Check sheet for the modelled part. Datum: model origin and axes. Units: mm. A direction names the side the tool comes from. Round coordinates to 2 decimals unless told otherwise and drop trailing zeros. Loops run counter-clockwise (first coordinate to the right, second up) from the corner with the lowest first, then second, coordinate; pieces in that order, holes last. Notation, with made-up numbers: (22.25, -22.5) - (59.25, -22.5) arc R24 cw to (59.25, 5.5) - close; hole circle Ø11 at (-17, 44). An arc over 180 degrees is marked (long way). Put each result on its own line as item: value. Start each with the question number.
Item 1: Gauge pin test, flat ends, axial feed: pin 1 Ø0.8 at (x, z) = (4, 97.5) entering from +Y; pin 2 Ø0.8 at (x, z) = (-3.5, 152.5) entering from -Y; pin 3 Ø1.5 at (x, y) = (-7.5, -1.5) entering from +Z (1 decimal); pin 4 Ø1.6 at (x, z) = (0.5, 215.5) entering from -Y. Record the tip position at first contact, or that the pin passes through.
Item 2: Section check C-C, the plane z = 235. Give the number of separate pieces and of enclosed holes in the cut face, and give its area (3 significant figures).
Item 3: Material ranges on line 1 along X through (y, z) = (7, 236); line 2 along Y through (x, z) = (-8.25, 139), recorded low to high.
Item 4: Section check A-A, the plane x = 0. Record the cut outline in (y, z), and give its area (3 significant figures).
Item 5: Tool access check on faces 1 (the flat face through (3.5, 0, 143)), 2 (the flat face through (0, -3.5, 143)), 3 (the flat face through (0, -3, 0)). Record the directions out of +Z, -Z, +X, -X, +Y, -Y that give a thin tool (end or side, any length) a straight path to the whole face; none if there is none.
Item 6: Draft check along X on faces 4 (the flat face through (-3.5, 0, 143)), 5 (the flat face through (0, -3, 290)), 6 (the cylindrical face through (-0.54, 2.44, 142.97)), 7 (the flat face through (0, 3.5, 143)). Enter one of: pulls with the +X half, pulls with the -X half, needs draft (parallel to the pull), parting line crosses it, or undercut.
Autodesk Inventor part; units mm, degrees
ref_plane "Начальная плоскость" through (0, 0, 0) normal (0, 0, 1) x (1, 0, 0)
ref_plane "Конечная плоскость" through (0, 0, 290) normal (0, 0, 1) x (1, 0, 0)
ref_plane "YZ Plane" through (0, 0, 0) normal (1, 0, 0) x (0, 1, 0)
ref_plane "Начальная плоскость" through (0, 0, 0) normal (0, 0, 1) x (1, 0, 0)
ref_plane "Конечная плоскость" through (0, 0, 290) normal (0, 0, 1) x (1, 0, 0)
sketch "Эскиз" plane through (0, 0, 0) normal (0, 0, 1) x (1, 0, 0)
  line L0 (-14.4349, 0) -> (14.4349, 0)
  line L1 (0, -14) -> (0, 14)
  line L2 (0, 0) -> (7.5, 7.5) construction
  circle A0 centre (7.5, 7.5) radius 1.65 construction
  line L3 (5.85, 9.15) -> (9.15, 9.15)
  line L4 (9.15, 9.15) -> (9.15, 5.85)
  line L5 (9.15, 5.85) -> (5.85, 5.85)
  line L6 (5.85, 5.85) -> (5.85, 9.15)
  line L7 (3.235, 8.1636) -> (4.72, 9.9636)
  line L8 (4.7971, 10) -> (8.5, 10)
  line L9 (3.3121, 8) -> (4.95, 8)
  line L10 (4.95, 8) -> (4.95, 5.7985)
  line L11 (4.95, 5.7985) -> (2.6515, 3.5)
  line L12 (0, 3.5) -> (2.6515, 3.5)
  circle A1 centre (0, 0) radius 2.5
  line L13 (8.1636, 3.235) -> (9.9636, 4.72)
  line L14 (10, 4.7971) -> (10, 8.5)
  line L15 (8, 3.3121) -> (8, 4.95)
  line L16 (8, 4.95) -> (5.7985, 4.95)
  line L17 (5.7985, 4.95) -> (3.5, 2.6515)
  line L18 (3.5, 0) -> (3.5, 2.6515)
  arc A2 (10, 8.5) -> (8.5, 10) centre (8.5, 8.5) ccw
  line L19 (0, 0) -> (-7.5, 7.5) construction
  circle A3 centre (-7.5, 7.5) radius 1.65 construction
  line L20 (-5.85, 9.15) -> (-9.15, 9.15)
  line L21 (-9.15, 9.15) -> (-9.15, 5.85)
  line L22 (-9.15, 5.85) -> (-5.85, 5.85)
  line L23 (-5.85, 5.85) -> (-5.85, 9.15)
  line L24 (-3.235, 8.1636) -> (-4.72, 9.9636)
  line L25 (-4.7971, 10) -> (-8.5, 10)
  line L26 (-3.3121, 8) -> (-4.95, 8)
  line L27 (-4.95, 8) -> (-4.95, 5.7985)
  line L28 (-4.95, 5.7985) -> (-2.6515, 3.5)
  line L29 (0, 3.5) -> (-2.6515, 3.5)
  line L30 (-3.5, 0) -> (-3.5, 2.6515)
  line L31 (-5.7985, 4.95) -> (-3.5, 2.6515)
  line L32 (-8, 4.95) -> (-5.7985, 4.95)
  line L33 (-8, 3.3121) -> (-8, 4.95)
  line L34 (-8.1636, 3.235) -> (-9.9636, 4.72)
  line L35 (-10, 4.7971) -> (-10, 8.5)
  arc A4 (-8.5, 10) -> (-10, 8.5) centre (-8.5, 8.5) ccw
  line L36 (0, 14) -> (0, -14)
  line L37 (0, 0) -> (7.5, -7.5) construction
  circle A5 centre (7.5, -7.5) radius 1.65 construction
  line L38 (5.85, -9.15) -> (9.15, -9.15)
  line L39 (9.15, -9.15) -> (9.15, -5.85)
  line L40 (9.15, -5.85) -> (5.85, -5.85)
  line L41 (5.85, -5.85) -> (5.85, -9.15)
  line L42 (3.235, -8.1636) -> (4.72, -9.9636)
  line L43 (4.7971, -10) -> (8.5, -10)
  line L44 (3.3121, -8) -> (4.95, -8)
  line L45 (4.95, -8) -> (4.95, -5.7985)
  line L46 (4.95, -5.7985) -> (2.6515, -3.5)
  line L47 (0, -3.5) -> (2.6515, -3.5)
  line L48 (3.5, 0) -> (3.5, -2.6515)
  line L49 (5.7985, -4.95) -> (3.5, -2.6515)
  line L50 (8, -4.95) -> (5.7985, -4.95)
  line L51 (8, -3.3121) -> (8, -4.95)
  line L52 (8.1636, -3.235) -> (9.9636, -4.72)
  line L53 (10, -4.7971) -> (10, -8.5)
  arc A6 (8.5, -10) -> (10, -8.5) centre (8.5, -8.5) ccw
  line L54 (0, 0) -> (-7.5, -7.5) construction
  line L55 (-4.95, -8) -> (-4.95, -5.7985)
  line L56 (-3.3121, -8) -> (-4.95, -8)
  line L57 (-5.7985, -4.95) -> (-3.5, -2.6515)
  line L58 (-4.95, -5.7985) -> (-2.6515, -3.5)
  line L59 (-3.5, 0) -> (-3.5, -2.6515)
  line L60 (0, -3.5) -> (-2.6515, -3.5)
  circle A7 centre (-7.5, -7.5) radius 1.65 construction
  line L61 (-5.85, -5.85) -> (-5.85, -9.15)
  line L62 (-5.85, -9.15) -> (-9.15, -9.15)
  line L63 (-9.15, -9.15) -> (-9.15, -5.85)
  line L64 (-9.15, -5.85) -> (-5.85, -5.85)
  line L65 (-3.235, -8.1636) -> (-4.72, -9.9636)
  line L66 (-8, -4.95) -> (-5.7985, -4.95)
  line L67 (-8, -3.3121) -> (-8, -4.95)
  line L68 (-8.1636, -3.235) -> (-9.9636, -4.72)
  line L69 (-4.7971, -10) -> (-8.5, -10)
  line L70 (-10, -4.7971) -> (-10, -8.5)
  arc A8 (-10, -8.5) -> (-8.5, -10) centre (-8.5, -8.5) ccw
  arc A9 (3.235, 8.1636) -> (3.3121, 8) centre (3.3121, 8.1) ccw
  arc A10 (4.7971, 10) -> (4.72, 9.9636) centre (4.7971, 9.9) ccw
  arc A11 (8, 3.3121) -> (8.1636, 3.235) centre (8.1, 3.3121) ccw
  arc A12 (9.9636, 4.72) -> (10, 4.7971) centre (9.9, 4.7971) ccw
  arc A13 (-3.3121, 8) -> (-3.235, 8.1636) centre (-3.3121, 8.1) ccw
  arc A14 (-4.72, 9.9636) -> (-4.7971, 10) centre (-4.7971, 9.9) ccw
  arc A15 (-8.1636, 3.235) -> (-8, 3.3121) centre (-8.1, 3.3121) ccw
  arc A16 (-10, 4.7971) -> (-9.9636, 4.72) centre (-9.9, 4.7971) ccw
  arc A17 (-8, -3.3121) -> (-8.1636, -3.235) centre (-8.1, -3.3121) ccw
  arc A18 (-9.9636, -4.72) -> (-10, -4.7971) centre (-9.9, -4.7971) ccw
  arc A19 (-3.235, -8.1636) -> (-3.3121, -8) centre (-3.3121, -8.1) ccw
  arc A20 (-4.7971, -10) -> (-4.72, -9.9636) centre (-4.7971, -9.9) ccw
  arc A21 (4.72, -9.9636) -> (4.7971, -10) centre (4.7971, -9.9) ccw
  arc A22 (3.3121, -8) -> (3.235, -8.1636) centre (3.3121, -8.1) ccw
  arc A23 (8.1636, -3.235) -> (8, -3.3121) centre (8.1, -3.3121) ccw
  arc A24 (10, -4.7971) -> (9.9636, -4.72) centre (9.9, -4.7971) ccw
  point P0 (3.1, 8)
  point P1 (4.75, 10)
  point P2 (7.5, 9.15)
  point P3 (8, 3.1)
  point P4 (10, 4.75)
  point P5 (7.5, 5.85)
  point P6 (9.15, 7.5)
  point P7 (-3.1, 8)
  point P8 (-4.75, 10)
  point P9 (-7.5, 9.15)
  point P10 (-8, 3.1)
  point P11 (-10, 4.75)
  point P12 (-7.5, 5.85)
  point P13 (-9.15, 7.5)
  point P14 (3.1, -8)
  point P15 (4.75, -10)
  point P16 (7.5, -9.15)
  point P17 (8, -3.1)
  point P18 (10, -4.75)
  point P19 (7.5, -5.85)
  point P20 (9.15, -7.5)
  point P21 (-3.1, -8)
  point P22 (-7.5, -5.85)
  point P23 (-7.5, -9.15)
  point P24 (-9.15, -7.5)
  point P25 (-4.75, -10)
  point P26 (-8, -3.1)
  point P27 (-10, -4.75)
  dimension "d0" = 45
  dimension "d1" = 3.3
  dimension "d2" = 1.5
  dimension "d3" = 1.2
  dimension "d4" = 5
  dimension "d5" = 6.5
  dimension "d6" = 15
  dimension "d7" = 20
  dimension "d8" = 9.9
  dimension "d9" = 9.5
  dimension "d10" = 6.2
  dimension "d11" = 2
  dimension "d18" = 0.1
  dimension "d19" = 0.1
extrude "Тело" add sketch "Эскиз" along normal up to surface (290 mm away) from surface at 0 contours A1 L1 L12 L11 L10 L9 A9 L7 A10 L8 A2 L14 A12 L13 A11 L15 L16 L17 L18 L0 | L0 L48 L49 L50 L51 A23 L52 A24 L53 A6 L43 A21 L42 A22 L44 L45 L46 L47 L1 A1 | A1 L0 L30 L31 L32 L33 A15 L34 A16 L35 A4 L25 A14 L24 A13 L26 L27 L28 L29 L1 | L1 L60 L58 L55 L56 A19 L65 A20 L69 A8 L70 A18 L68 A17 L67 L66 L57 L59 L0 A1
sketch "Эскиз2" plane through (0, 0, 0) normal (0, 0, 1) x (1, 0, 0)
  line L0 (0, 0) -> (10, 0)
ref_plane "РабПлоскость3" through (0, 0, 0) normal (0, -1, 0) x (1, 0, 0)
sketch "Эскиз3" plane through (0, 0, 0) normal (0, -1, 0) x (1, 0, 0)
  line L0 (-2, 0) -> (12, 0)
  line L1 (-2, 290) -> (12, 290)
  dimension "d25" = 290
equation "\"G_OFFSET_START\" = 0"
equation "\"G_OFFSET_END\" = 0"
properties part number "короткая палка"
Check result:
1. pin 1: y = 9.58
1. pin 2: y = -8.97
1. pin 3: through
1. pin 4: y = -3.5
2. separate pieces: 1
2. enclosed holes: 5
2. area: 115 mm²
3. line 1: -10 to -9.15, -5.85 to -4.95, 4.95 to 5.85, 9.15 to 10
3. line 2: -10 to -9.15, -5.85 to -3.31, 3.31 to 5.85, 9.15 to 10
4. outline: (-3.5, 0) - (-2.5, 0) - (-2.5, 290) - (-3.5, 290) - close; (2.5, 0) - (3.5, 0) - (3.5, 290) - (2.5, 290) - close
4. area: 580 mm²
5. face 1: +Z, -Z, +X
5. face 2: +Z, -Z, -Y
5. face 3: -Z, +X, -X, +Y, -Y
6. face 4: pulls with the -X half
6. face 5: needs draft
6. face 6: undercut
6. face 7: undercut
